Verification items for the finished model (mm, model axes). Round coordinates to 2 decimals unless told otherwise and drop trailing zeros. Write each loop counter-clockwise with the first axis right and the second up, starting at its lowest first coordinate (ties: lowest second). Pieces come first, ordered by that corner, then holes. Notation, with made-up numbers: M 31,43 L 61,43 A16 cw 61,73 Z; hole C 33,-17.5 d11. An arc over 180 degrees is marked long. One line per question, with ' | ' between items.
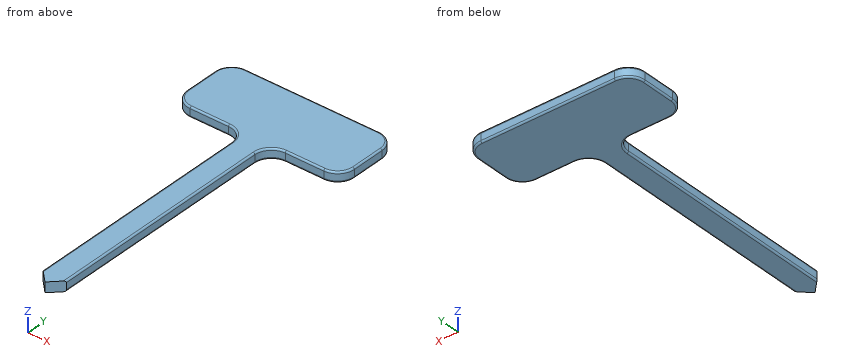
from build123d import *

# Parameters (mm, degrees)
F0_W        = 7
F0_H        = 80
F1_DEPTH    = 3
F2_R        = 5
F3_T1_DEPTH = 39.0035618315
F4_R        = 0.5


# Not quite as in the source:
# - a fillet or chamfer that OpenCascade refuses, or shapes differently, is made with other operations: its cross-section is extruded or revolved along the edge and cut away or added


with BuildPart() as f1:
    # F0 (on Top) → F1 (new body)
    with BuildSketch(Plane.XY):
        Polygon((-25, 73.9269424736), (-25, 53.9269424736), (-3.5, 53.9269424736), (3.5, 53.9269424736), (25, 53.9269424736), (25, 73.9269424736), align=None)
        with Locations((0, 13.9269424736)):
            Rectangle(F0_W, F0_H)
    extrude(amount=F1_DEPTH)

    # F2
    f2_edges = [f1.edges().sort_by_distance(p)[0] for p in [
        (-25, 73.926942, 1.5),
        (25, 73.926942, 1.5),
        (25, 53.926942, 1.5),
        (3.5, 53.926942, 1.5),
        (-3.5, 53.926942, 1.5),
        (-25, 53.926942, 1.5),
    ]]
    fillet(f2_edges, radius=F2_R)

    # F3: chamfer of 7 on 2 edges, made by hand

    # F3_s2 → F3_t1 (cut)
    with BuildSketch(Plane.XY.offset(-18.0017809158)):
        Polygon((-3.5, -19.0730575264), (3.5, -26.0730575264), (-3.5, -26.0730575264), align=None)
        Polygon((-3.5, -26.0730575264), (3.5, -19.0730575264), (3.5, -26.0730575264), align=None)
    extrude(amount=F3_T1_DEPTH, mode=Mode.SUBTRACT)

    # F4
    f4_edges = [f1.edges().sort_by_distance(p)[0] for p in [
        (-3.5, 14.926942, 3),
        (-3.5, 14.926942, 0),
    ]]
    fillet(f4_edges, radius=F4_R)


solid = f1.part
1. Section check C-C, the plane z = 1.75. Record the cut outline in (x, y), then the cut area to 3 significant figures.
Results:
outline: M -25,58.93 A5 ccw -20,53.93 L -8.5,53.93 A5 cw -3.5,48.93 L -3.5,-19.07 L 0,-22.57 L 3.5,-19.07 L 3.5,48.93 A5 cw 8.5,53.93 L 20,53.93 A5 ccw 25,58.93 L 25,68.93 A5 ccw 20,73.93 L -20,73.93 A5 ccw -25,68.93 Z | area: 1,510 mm2
2. Go/stop test with flat-tipped pins: P1, Ø1, axis at y = 27, z = 1, coming from the -X side; P2, Ø0.6, axis at x = -11.5, z = 1.5, coming from the -Y side; P3, Ø1, axis at y = -1, z = 1.5, coming from the +X side. Record where each tip stops, or that it passes through.
Results:
P1: stops at x = -3.5 | P2: stops at y = 53.93 | P3: stops at x = 3.5
3. Section check B-B, the plane y = -7.5. Record the cut outline in (x, z), then the cut area to 3 significant figures.
Results:
outline: M -3.5,0.5 A0.5 ccw -3,0 L 3,0 A0.5 ccw 3.5,0.5 L 3.5,2.5 A0.5 ccw 3,3 L -3,3 A0.5 ccw -3.5,2.5 Z | area: 20.8 mm2
4. Section check A-A, the plane x = 13. Record the cut outline in (y, z).
Results:
outline: M 53.93,0.5 A0.5 ccw 54.43,0 L 73.43,0 A0.5 ccw 73.93,0.5 L 73.93,2.5 A0.5 ccw 73.43,3 L 54.43,3 A0.5 ccw 53.93,2.5 Z
5. Thickness scan on line 1 (Y direction, x = 16.5, z = 2.3); line 2 (Y direction, x = 3, z = 1); line 3 (X direction, y = 8, z = 1.2). Record the ranges inside material, lowest first.
Results:
line 1: y = 53.93 to 73.93 | line 2: y = -19.57 to 73.93 | line 3: x = -3.5 to 3.5
